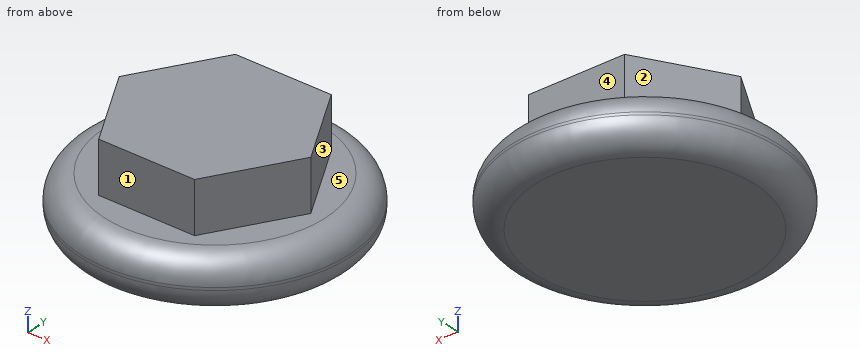
from build123d import *

# Parameters (mm, degrees)
F0_R     = 12.7
F1_DEPTH = 4.826
F3_DEPTH = 4.826
F4_R     = 2.286
F5_R     = 2.286


with BuildPart() as f1:
    # F0 (on Top) → F1 (new body)
    with BuildSketch(Plane.XY):
        Circle(F0_R)
    extrude(amount=F1_DEPTH)

    # F2 (on face) → F3 (join)
    with BuildSketch(Plane.XY.offset(4.826)):
        Polygon((4.582718, 7.9375), (-4.582718, 7.9375), (-9.165436, 0), (-4.582718, -7.9375), (4.582718, -7.9375), (9.165436, 0), align=None)
    extrude(amount=F3_DEPTH)

    # F4
    f4_edges = [f1.edges().sort_by_distance(p)[0] for p in [
        (-12.7, 0, 4.826),
    ]]
    fillet(f4_edges, radius=F4_R)

    # F5
    f5_edges = [f1.edges().sort_by_distance(p)[0] for p in [
        (-12.7, 0, 0),
    ]]
    fillet(f5_edges, radius=F5_R)


solid = f1.part
Model file for the job. Use its own axes, mm. Face numbers are marked on the shaded views. A direction names the side the tool comes from. Give positions to 0.01 mm unless a question says otherwise; leave off trailing zeros. Order: outer loops, then holes, each group sorted by start corner. A loop starts at its lowest first (then second) coordinate and runs counter-clockwise, first axis right, second up. Notation, with made-up numbers: (22.5, -21) -> (60.5, -21) arc R16 cw to (60.5, -9) -> close; hole circle Ø8 at (44, 18.5). An arc over 180 degrees is marked (long way). Use CSV: the item, a comma, the result in double quotes.
1. 3-axis set-ups, long thin cutter, end or side, ignore diameter. For the marked faces 1, 2, 3, 4 and 5: which of +Z, -Z, +X, -X, +Y, -Y reach the whole face in a straight line?
Outcome:
face 1,"+Z, +X, -X, -Y"
face 2,"+Z, -X, +Y"
face 3,"+Z, +X, +Y"
face 4,"+Z, +X, -X, +Y"
face 5,"+Z"
2. Drill centre lines: line 1 along Z through (x, y) = (8.5, 4.75); line 2 along Y through (x, z) = (0.75, 5.75); line 3 along Y through (x, z) = (4.75, 8.5). Where is each one in solid material? Low to high. Write a range as from..to.
Outcome:
line 1,"0..4.83"
line 2,"-7.94..7.94"
line 3,"-7.65..7.65"
3. Band-saw the part on B-B, the plane x = 0. Give the cut face in (y, z).
Outcome:
outline,"(-12.7, 2.29) arc R2.29 ccw to (-10.41, 0) -> (10.41, 0) arc R2.29 ccw to (12.7, 2.29) -> (12.7, 2.54) arc R2.29 ccw to (10.41, 4.83) -> (7.94, 4.83) -> (7.94, 9.65) -> (-7.94, 9.65) -> (-7.94, 4.83) -> (-10.41, 4.83) arc R2.29 ccw to (-12.7, 2.54) -> close"
4. Drop flat-ended pins along their axis: pin 1 (1 mm diameter, centred on y = -3, z = 4, fed in from -X); pin 2 (4 mm diameter, centred on x = 0, z = 7.5, fed in from +Y); pin 3 (1 mm diameter, centred on y = -6, z = 8.5, fed in from -X). Give the stop position or say it passes through.
Outcome:
pin 1,"x = -12.15"
pin 2,"y = 7.94"
pin 3,"x = -5.99"
5. Band-saw the part on A-A, the plane z = 5.5. Give the cut face in (x, y), then the cut area to 3 significant figures.
Outcome:
outline,"(-9.17, 0) -> (-4.58, -7.94) -> (4.58, -7.94) -> (9.17, 0) -> (4.58, 7.94) -> (-4.58, 7.94) -> close"
area,"218 mm²"
